For this review, use the dimensioned drawing (mm, ordinates from the lowest corner) and the shaded views. Round coordinates to 2 decimals unless told otherwise and drop trailing zeros. Order: outer loops, then holes, each group sorted by start corner. A loop starts at its lowest first (then second) coordinate and runs counter-clockwise, first axis right, second up. Notation, with made-up numbers: M -34.75,81.25 L 13.25,81.25 A13 ccw 13.25,105.25 Z; hole C 19,27 d7. An arc over 180 degrees is marked long. Put each result on its own line as item: value.
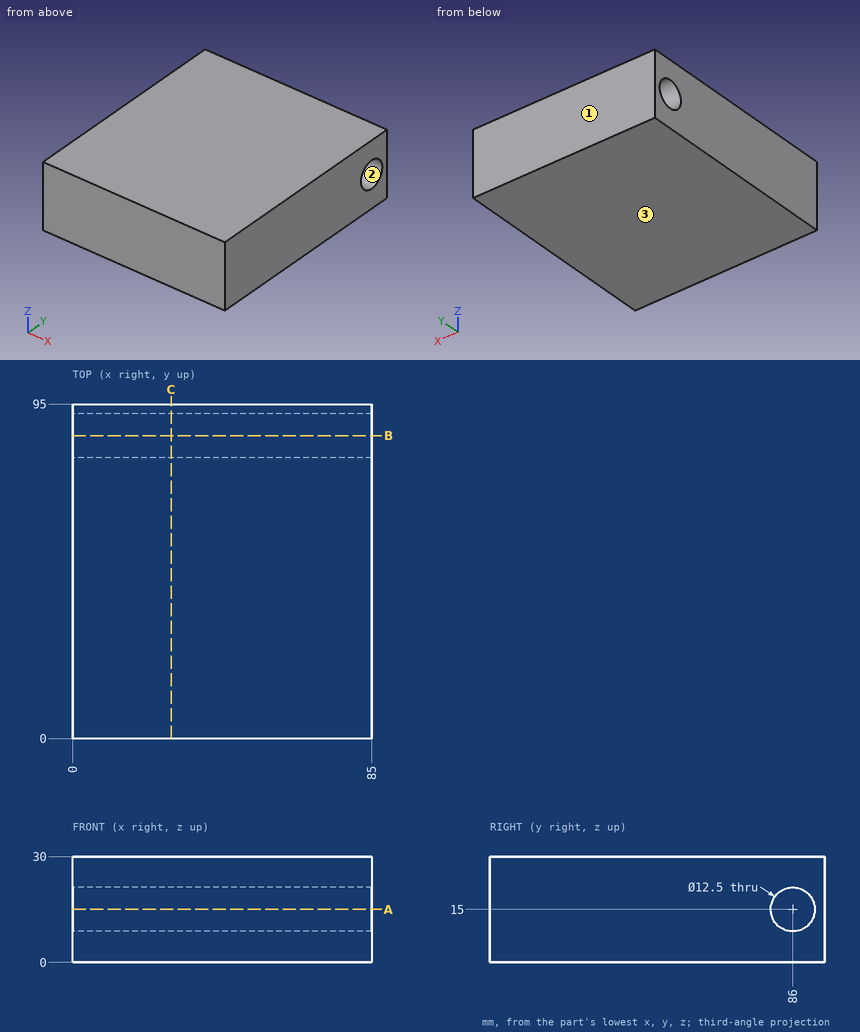
(1) Insertion check: pin 1 Ø4 at (y, z) = (63, 6) entering from -X. The pin has a flat end and moves straight along its axis. Give the tip position at first contact, or say it passes through.
A:
pin 1: stops at x = 0
(2) Add section C-C on x = 28. Give the boundary of the cut face in (y, z), then the cut area to 3 significant figures.
A:
outline: M 0,0 L 95,0 L 95,30 L 0,30 Z; hole C 86,15 d12.5
area: 2,730 mm2
(3) Add section A-A on z = 15. Give the boundary of the cut face in (x, y), then the cut area to 3 significant figures.
A:
outline: M 0,0 L 85,0 L 85,79.75 L 0,79.75 Z; M 0,92.25 L 85,92.25 L 85,95 L 0,95 Z
area: 7,010 mm2
(4) Add section B-B on y = 86. Give the boundary of the cut face in (x, z), then the cut area to 3 significant figures.
A:
outline: M 0,0 L 85,0 L 85,8.75 L 0,8.75 Z; M 0,21.25 L 85,21.25 L 85,30 L 0,30 Z
area: 1,490 mm2
(5) Draft analysis for pull direction Z (two halves, no side actions). For the marked faces 1, 2 and 3, state which applies: released by +Z, released by -Z, zero draft, split by the parting line, or undercut.
A:
face 1: zero draft
face 2: undercut
face 3: released by -Z
(6) To check wall thickness, follow L1, parallel to Y at x = 37.5, z = 15; L2, parallel to Z at x = 40, y = 86; L3, parallel to Y at x = 61, z = 20.75. State the ranges of each line that lie inside material, in increasing order.
A:
L1: y = 0 to 79.75, 92.25 to 95
L2: z = 0 to 8.75, 21.25 to 30
L3: y = 0 to 83.55, 88.45 to 95
